Autodesk Fusion 360 part; units mm, degrees
sketch "Sketch1" plane through (0, 0, 0) normal (0, 0, 1) x (1, 0, 0)
  circle A0 centre (0, 0) radius 25.4
  circle A1 centre (0, 0) radius 19.05
  circle A2 centre (0, 0) radius 22.225 construction
  line L0 (0, 0) -> (0, 25.4) construction
  point P0 (0, 22.225)
  dimension "d1" = 50.8
  dimension "d2" = 38.1
  dimension "d5" = 44.45
extrude "Extrude1" add sketch "Sketch1" along normal blind 25.4
hole "Hole1" at (0, 0, 0) direction (0, 0, -1) diameter 3.4163 depth 25.4 tip angle 118
pattern_circular "C-Pattern1" count 3 over 360 about axis through (0, 0, 0) along (0, 0, 1) of "Hole1"
sketch "Sketch3" plane through (0, 0, 0) normal (0, 1, 0) x (1, 0, 0)
  line L0 (-25.4, -25.4) -> (25.4, -25.4)
  line L1 (-25.4, 0) -> (25.4, 0)
  line L2 (0, 0) -> (0, -12.7) construction
  line L3 (0, -12.7) -> (0, -25.4) construction
  circle A0 centre (0, -12.7) radius 3.175
  point P0 (0, -12.7)
  dimension "d12" = 6.35
extrude "Extrude2" cut sketch "Sketch3" against normal blind 25.4
Part model, mm, in its own coordinate system. Coordinates: 2 decimals unless noted, no trailing zeros. Order: outer loops, then holes, each group sorted by start corner. A loop starts at its lowest first (then second) coordinate and runs counter-clockwise, first axis right, second up. Notation, with made-up numbers: (-27, -38.75) - (24, -38.75) arc R24 ccw to (24, -16.75) - close; hole circle Ø1 at (42.25, 34.5). An arc over 180 degrees is marked (long way). Return JSON: item names as keys, results as strings. Group by question number.
Item 1: Cut at B-B (x = 10). List the corners of the cut face in (y, z).
Item 2: Pull direction X, two halves, no side cores. Call faces 1 (the face through (-5.506, 24.796, 12.522)), 2 (the face through (-0.69, -22.05, 15.8)), 3 (the face through (4, 19, 0)): pulls with the +X half, pulls with the -X half, needs draft (parallel to the pull), parting line crosses it, or undercut.
Item 3: Cut at A-A (y = 0). List the corners of the cut face in (x, z), plus the area to 3 significant figures.
Item 4: Drill centre lines: probe 1 along Z at (x, y) = (0, -20) (3 decimals); probe 2 along X at (y, z) = (0.5, 7.5); probe 3 along Y at (x, z) = (0, 20.75). Where is each one in solid material? Low to high. Write a range as from..to.
Item 5: Cut at C-C (x = 0). List the corners of the cut face in (y, z) (3 decimals), plus the area to 3 significant figures.
Item 6: Cut at D-D (z = 7.5). List the corners of the cut face in (x, y).
Item 7: Pin check, flat tips, straight feed: pin 1 (1 mm diameter, centred on x = -8.5, z = 22.5, fed in from +Y); pin 2 (1.5 mm diameter, centred on x = -6, z = 14.5, fed in from +Y); pin 3 (1.5 mm diameter, centred on x = 2.5, z = 16.5, fed in from -Y). Stop position of each tip, or through.
Check values:
{
 "1": {"outline": "(-23.35, 0) - (-16.21, 0) - (-16.21, 25.4) - (-23.35, 25.4) - close; (16.21, 0) - (23.35, 0) - (23.35, 25.4) - (16.21, 25.4) - close"},
 "2": {"face 1": "parting line crosses it", "face 2": "undercut", "face 3": "needs draft"},
 "3": {"outline": "(-25.4, 0) - (-19.05, 0) - (-19.05, 25.4) - (-25.4, 25.4) - close; (19.05, 0) - (25.4, 0) - (25.4, 25.4) - (19.05, 25.4) - close", "area": "323 mm2"},
 "4": {"probe 1": "z = 0..9.525, 15.875..25.4", "probe 2": "x = -25.4..-19.04, 19.04..25.4", "probe 3": "y = -25.4..-19.05, 19.05..25.4"},
 "5": {"outline": "(-25.4, 0) - (-19.05, 0) - (-19.05, 9.525) - (-25.4, 9.525) - close; (-25.4, 15.875) - (-19.05, 15.875) - (-19.05, 25.4) - (-25.4, 25.4) - close; (19.05, 0) - (25.4, 0) - (25.4, 25.4) - (19.05, 25.4) - close", "area": "282 mm2"},
 "6": {"outline": "circle Ø50.8 at (0, 0); hole circle Ø38.1 at (0, 0)"},
 "7": {"pin 1": "stops at y = 24.11", "pin 2": "stops at y = 24.85", "pin 3": "stops at y = -25.34"}
}
